from build123d import *

# Parameters (mm, degrees)
F1_DEPTH = 2


with BuildPart() as f1:
    # F0 (on Top) → F1 (new body)
    with BuildSketch(Plane.XY):
        with BuildLine():
            add(Edge.make_bspline(
                [(8.6748898029, 5.6916326284), (8.6487335954, 5.4451622036), (8.9050139712, 4.6956597308), (10.3461055042, 4.2046193666), (12.0542033217, 4.0215565005), (12.7291959786, 4.1737857422), (13.0162881687, 4.2385328561)],
                knots=[0.1411262008, 0.1411262008, 0.1411262008, 0.1411262008, 0.3215319836, 0.5569055766, 0.8115402483, 1, 1, 1, 1], degree=3))
            Line((8.6748898029, 5.6916326284), (-37.6118458807, 5.7461173274))
            add(Edge.make_bspline(
                [(-37.6118458807, 5.7461173274), (-40.5734612696, 5.5933859506), (-46.0074223206, 5.0041541834), (-53.904567956, 3.8883420379), (-60.4349233984, 2.5040791618), (-65.0644995905, 1.4725007887), (-68.5725675359, 0.5033486653), (-70.3945532441, 0)],
                knots=[0.3193249377, 0.3193249377, 0.3193249377, 0.3193249377, 0.4741629094, 0.6243096755, 0.7604296541, 0.8755743181, 1, 1, 1, 1], degree=3))
            add(Edge.make_bspline(
                [(-37.6118458807, -5.7461173274), (-40.5734612696, -5.5933859506), (-46.0074223206, -5.0041541834), (-53.904567956, -3.8883420379), (-60.4349233984, -2.5040791618), (-65.0644995905, -1.4725007887), (-68.5725675359, -0.5033486653), (-70.3945532441, 0)],
                knots=[0.3193249377, 0.3193249377, 0.3193249377, 0.3193249377, 0.4741629094, 0.6243096755, 0.7604296541, 0.8755743181, 1, 1, 1, 1], degree=3))
            Line((-37.6118458807, -5.7461173274), (8.6748898029, -5.6916326284))
            add(Edge.make_bspline(
                [(8.6748898029, -5.6916326284), (8.6487335954, -5.4451622036), (8.9050139712, -4.6956597308), (10.3461055042, -4.2046193666), (12.0542033217, -4.0215565005), (12.7291959786, -4.1737857422), (13.0162881687, -4.2385328561)],
                knots=[0.1411262008, 0.1411262008, 0.1411262008, 0.1411262008, 0.3215319836, 0.5569055766, 0.8115402483, 1, 1, 1, 1], degree=3))
            add(Edge.make_bspline(
                [(13.0162881687, -4.2385328561), (13.5212335751, -6.8386267952), (14.5412711945, -12.0910631935), (12.3149675559, -21.397985611), (12.0986721053, -21.9763078704), (12.0552927256, -22.0922939479)],
                knots=[0, 0, 0, 0, 0.4393662274, 0.887561457, 1, 1, 1, 1], degree=3))
            Line((12.0552927256, -22.0922939479), (15.5880060047, -25.4827160388))
            Line((15.5880060047, -25.4827160388), (19.0819334239, -22.1619550139))
            add(Edge.make_bspline(
                [(19.0819334239, -22.1619550139), (18.6267322874, -20.294252499), (17.7386984759, -16.6506258682), (17.2606082512, -11.5156236051), (17.7756044656, -7.4243914642), (18.0465597659, -5.2718687803)],
                knots=[0, 0, 0, 0, 0.3326029965, 0.6488619712, 1, 1, 1, 1], degree=3))
            Line((18.0465597659, -5.2718687803), (18.0465597659, -4.1968291625))
            Line((18.0465597659, -4.1968291625), (18.2820949703, -4.1968291625))
            add(Edge.make_bspline(
                [(18.2820949703, -4.1968291625), (18.6553641024, -4.0763285269), (19.4680558232, -3.8139712612), (20.4982628837, -4.1457607251), (21.0552960634, -4.3251593597)],
                knots=[0, 0, 0, 0, 0.4592997844, 1, 1, 1, 1], degree=3))
            add(Edge.make_bspline(
                [(21.0552960634, -4.3251593597), (21.2135892272, -4.39182334), (21.5216440654, -4.5215583278), (21.8009874785, -4.3894057062), (21.9367910177, -4.3251593597)],
                knots=[0, 0, 0, 0, 0.5138473549, 1, 1, 1, 1], degree=3))
            Line((21.9367910177, -4.3251593597), (27.6336535588, -4.5601242409))
            add(Edge.make_bspline(
                [(27.6336535588, -4.5601242409), (28.2535762385, -4.5515479471), (28.8568336912, -4.5327320205), (29.4600911438, -4.5139160939)],
                knots=[0.7364720785, 0.7364720785, 0.7364720785, 0.7364720785, 1, 1, 1, 1], degree=3))
            add(Edge.make_bspline(
                [(29.4600911438, -4.5139160939), (29.602363452, -4.5612346279), (29.7446357601, -4.6085531619), (29.9036486376, -4.6537493056)],
                knots=[0, 0, 0, 0, 0.1239808677, 0.1239808677, 0.1239808677, 0.1239808677], degree=3))
            Line((29.9036486376, -4.6537493056), (52.4882189929, -5.5852411315))
            add(Edge.make_bspline(
                [(52.4882189929, -5.5852411315), (53.3910924323, -5.3930971357), (56.8432596926, -3.8943500714), (57.5901163978, -3.1391917956), (57.8616410494, -2.8646490537)],
                knots=[0.1940769563, 0.1940769563, 0.1940769563, 0.1940769563, 0.7070013938, 1, 1, 1, 1], degree=3))
            ThreePointArc((57.8616410494, -2.8646490537), (58.6164496784, 0), (57.8616410494, 2.8646490537))
            add(Edge.make_bspline(
                [(52.4882189929, 5.5852411315), (53.3910924323, 5.3930971357), (56.8432596926, 3.8943500714), (57.5901163978, 3.1391917956), (57.8616410494, 2.8646490537)],
                knots=[0.1940769563, 0.1940769563, 0.1940769563, 0.1940769563, 0.7070013938, 1, 1, 1, 1], degree=3))
            Line((52.4882189929, 5.5852411315), (29.9036486376, 4.6537493056))
            add(Edge.make_bspline(
                [(29.4600911438, 4.5139160939), (29.602363452, 4.5612346279), (29.7446357601, 4.6085531619), (29.9036486376, 4.6537493056)],
                knots=[0, 0, 0, 0, 0.1239808677, 0.1239808677, 0.1239808677, 0.1239808677], degree=3))
            add(Edge.make_bspline(
                [(27.6336535588, 4.5601242409), (28.2535762385, 4.5515479471), (28.8568336912, 4.5327320205), (29.4600911438, 4.5139160939)],
                knots=[0.7364720785, 0.7364720785, 0.7364720785, 0.7364720785, 1, 1, 1, 1], degree=3))
            Line((27.6336535588, 4.5601242409), (21.9367910177, 4.3251593597))
            add(Edge.make_bspline(
                [(21.0552960634, 4.3251593597), (21.2135892272, 4.39182334), (21.5216440654, 4.5215583278), (21.8009874785, 4.3894057062), (21.9367910177, 4.3251593597)],
                knots=[0, 0, 0, 0, 0.5138473549, 1, 1, 1, 1], degree=3))
            add(Edge.make_bspline(
                [(18.2820949703, 4.1968291625), (18.6553641024, 4.0763285269), (19.4680558232, 3.8139712612), (20.4982628837, 4.1457607251), (21.0552960634, 4.3251593597)],
                knots=[0, 0, 0, 0, 0.4592997844, 1, 1, 1, 1], degree=3))
            Line((18.2820949703, 4.1968291625), (18.0465597659, 4.1968291625))
            Line((18.0465597659, 4.1968291625), (18.0465597659, 5.2718687803))
            add(Edge.make_bspline(
                [(19.0819334239, 22.1619550139), (18.6267322874, 20.294252499), (17.7386984759, 16.6506258682), (17.2606082512, 11.5156236051), (17.7756044656, 7.4243914642), (18.0465597659, 5.2718687803)],
                knots=[0, 0, 0, 0, 0.3326029965, 0.6488619712, 1, 1, 1, 1], degree=3))
            Line((19.0819334239, 22.1619550139), (15.5880060047, 25.4827160388))
            Line((15.5880060047, 25.4827160388), (12.0552927256, 22.0922939479))
            add(Edge.make_bspline(
                [(13.0162881687, 4.2385328561), (13.5212335751, 6.8386267952), (14.5412711945, 12.0910631935), (12.3149675559, 21.397985611), (12.0986721053, 21.9763078704), (12.0552927256, 22.0922939479)],
                knots=[0, 0, 0, 0, 0.4393662274, 0.887561457, 1, 1, 1, 1], degree=3))
        make_face()
    extrude(amount=F1_DEPTH)


solid = f1.part
Part model, mm, in its own coordinate system. Give positions to 0.01 mm unless a question says otherwise; leave off trailing zeros. Loops run counter-clockwise (first coordinate to the right, second up) from the corner with the lowest first, then second, coordinate; pieces in that order, holes last.
(1) Band-saw the part on B-B (x = -23.5). Write the cut outline in (y, z).
Return value:
outline: (-5.73, 0) - (5.73, 0) - (5.73, 2) - (-5.73, 2) - close
(2) Drill centre lines: line 1 along Y through (x, z) = (22.5, 1.4); line 2 along Y through (x, z) = (-15, 0.7); line 3 along X through (y, z) = (11, 1). Where is each one in solid material? Low to high.
Return value:
line 1: y = -4.35 to 4.35
line 2: y = -5.72 to 5.72
line 3: x = 13.85 to 17.48
(3) Pin check, flat tips, straight feed: pin 1 (0.9 mm diameter, centred on y = 5, z = 0.5, fed in from +X); pin 2 (0.5 mm diameter, centred on y = -4.5, z = 1.5, fed in from +X). Stop position of each tip, or through.
Return value:
pin 1: stops at x = 55.2
pin 2: stops at x = 55.83
(4) Band-saw the part on A-A (x = 36.5). Write the cut outline in (y, z), and give its area (3 significant figures).
Return value:
outline: (-4.93, 0) - (4.93, 0) - (4.93, 2) - (-4.93, 2) - close
area: 19.7 mm2
